Design review of the part built by this model. Coordinates are the model's own, in mm. A direction names the side the tool comes from. Coordinates: 2 decimals unless noted, no trailing zeros. Loops run counter-clockwise (first coordinate to the right, second up) from the corner with the lowest first, then second, coordinate; pieces in that order, holes last. Notation, with made-up numbers: (63, 44.5) -> (82, 44.5) arc R23 ccw to (82, 64.5) -> close; hole circle Ø5 at (-26.75, 74.5). An arc over 180 degrees is marked (long way). Use CSV: the item, a comma, the result in double quotes.
```python
from build123d import *

# Parameters (mm, degrees)
SKETCH1_R               = 40
SKETCH1_R_2             = 30
SKETCH1_R_3             = 3
BOSS_EXTRUDE1_DEPTH     = 18.5
CUT_EXTRUDE1_DEPTH      = 6.25
CUT_EXTRUDE1_DEPTH_BACK = 6.25
SKETCH2_R               = 42.5
SKETCH2_R_2             = 30


with BuildPart() as part:
    # Sketch1 → Boss-Extrude1 (new body)
    # profile 1 of 2: a face of its own
    with BuildSketch(Plane.XY):
        Circle(SKETCH1_R)
        Circle(SKETCH1_R_2, mode=Mode.SUBTRACT)
    # profile 2 of 2: a face of its own
    with BuildSketch(Plane.XY):
        Circle(SKETCH1_R_2)
        Circle(SKETCH1_R_3, mode=Mode.SUBTRACT)
    extrude(amount=BOSS_EXTRUDE1_DEPTH)

    # Sketch2 → Cut-Extrude1 (cut, two sides: drawn at the far end of the back side and taken through both)
    with BuildSketch(Plane.XY.offset(9.25).offset(-CUT_EXTRUDE1_DEPTH_BACK)):
        Circle(SKETCH2_R)
        Circle(SKETCH2_R_2, mode=Mode.SUBTRACT)
    extrude(amount=CUT_EXTRUDE1_DEPTH + CUT_EXTRUDE1_DEPTH_BACK, mode=Mode.SUBTRACT)


solid = part.part
```
Item 1: Add section C-C (z = 4). Give the boundary of the cut face in (x, y), then the cut area to 3 significant figures.
Checked values:
outline,"circle Ø60 at (0, 0); hole circle Ø6 at (0, 0)"
area,"2,800 mm^2"
Item 2: Clearance check with flat-ended pins moving along their axes: pin 1 (2 mm diameter, centred on y = 10, z = 2, fed in from +X); pin 2 (10 mm diameter, centred on y = 25.5, z = 15.5, fed in from -X); pin 3 (8 mm diameter, centred on y = -18.5, z = 6.5, fed in from +X). State where each tip first meets the part, or that it passes through.
Checked values:
pin 1,"x = 38.97"
pin 2,"x = -34.35"
pin 3,"x = 36.41"
Item 3: Draft analysis for pull direction Z (two halves, no side actions). For faces 3 (the face through (6, 30, 15.5)), 4 (the face through (8, 1, 18.5)), 5 (the face through (-29.97, 1.32, 9.16)), 6 (the face through (-8.67, -39.05, 1.48)), state which applies: pulls with the +Z half, pulls with the -Z half, needs draft (parallel to the pull), parting line crosses it, or undercut.
Checked values:
face 3,"undercut"
face 4,"pulls with the +Z half"
face 5,"undercut"
face 6,"needs draft"
Item 4: Add section D-D (y = -16). Give the boundary of the cut face in (x, z).
Checked values:
outline,"(-36.66, 0) -> (36.66, 0) -> (36.66, 3) -> (25.38, 3) -> (25.38, 15.5) -> (36.66, 15.5) -> (36.66, 18.5) -> (-36.66, 18.5) -> (-36.66, 15.5) -> (-25.38, 15.5) -> (-25.38, 3) -> (-36.66, 3) -> close"
Item 5: To check wall thickness, follow line 1 along Z through (x, y) = (12.5, 29); line 2 along Y through (x, z) = (0, 6.5); line 3 along Y through (x, z) = (-1, 12). State the ranges of each line that lie inside material, in increasing order.
Checked values:
line 1,"0 to 3, 15.5 to 18.5"
line 2,"-30 to -3, 3 to 30"
line 3,"-29.98 to -2.83, 2.83 to 29.98"
Item 6: Add section A-A (x = 0). Give the boundary of the cut face in (y, z), then the cut area to 3 significant figures.
Checked values:
outline,"(-40, 0) -> (-3, 0) -> (-3, 18.5) -> (-40, 18.5) -> (-40, 15.5) -> (-30, 15.5) -> (-30, 3) -> (-40, 3) -> close; (3, 0) -> (40, 0) -> (40, 3) -> (30, 3) -> (30, 15.5) -> (40, 15.5) -> (40, 18.5) -> (3, 18.5) -> close"
area,"1,120 mm^2"
Item 7: Machinability: for faces 1 (the face through (8, 1, 0)), 2 (the face through (6, 30, 3)), which of the approach directions +Z, -Z, +X, -X, +Y, -Y give a long, thin tool a straight path to every point of the face, cutting with its end or side? Answer none if there is none.
Checked values:
face 1,"-Z, +X, -X, +Y, -Y"
face 2,"none"
